Answer from the drawing. Dimensions are ordinates in mm from the lowest x, y and z of the part. Coordinates: 2 decimals unless noted, no trailing zeros. Order: outer loops, then holes, each group sorted by start corner. A loop starts at its lowest first (then second) coordinate and runs counter-clockwise, first axis right, second up. Notation, with made-up numbers: (35, -19) - (77, -19) arc R26 ccw to (77, 10) - close; hole circle Ø6 at (-33, 65). An arc over 180 degrees is marked (long way). Use a Markdown table: item, result. Add a question column.
Item 1: The part is cut by section A-A, the plane y = 63.5. Give the vertices of the cut face in (x, z), then the cut area to 3 significant figures.
Item 2: The part is cut by section B-B, the plane x = 416.5. Give the vertices of the cut face in (y, z), then the cut area to 3 significant figures.
Item 3: Find the intervals of material crossed by line 1 along Y through (x, z) = (1130, 64.5); line 2 along Z through (x, y) = (1079, 68.5); line 3 along Z through (x, y) = (1245.5, 66), in increasing order.
Item 4: Flat-ended cylindrical pins translate along their axes: P1, Ø4, axis at x = 621.5, z = 29.5, coming from the -Y side; P2, Ø5, axis at x = 978.5, y = 98.5, coming from the -Z side; P3, Ø10, axis at x = 702.5, y = 55.5, coming from the +Z side. Find the tip coordinate at first contact, or state that the pin passes through.
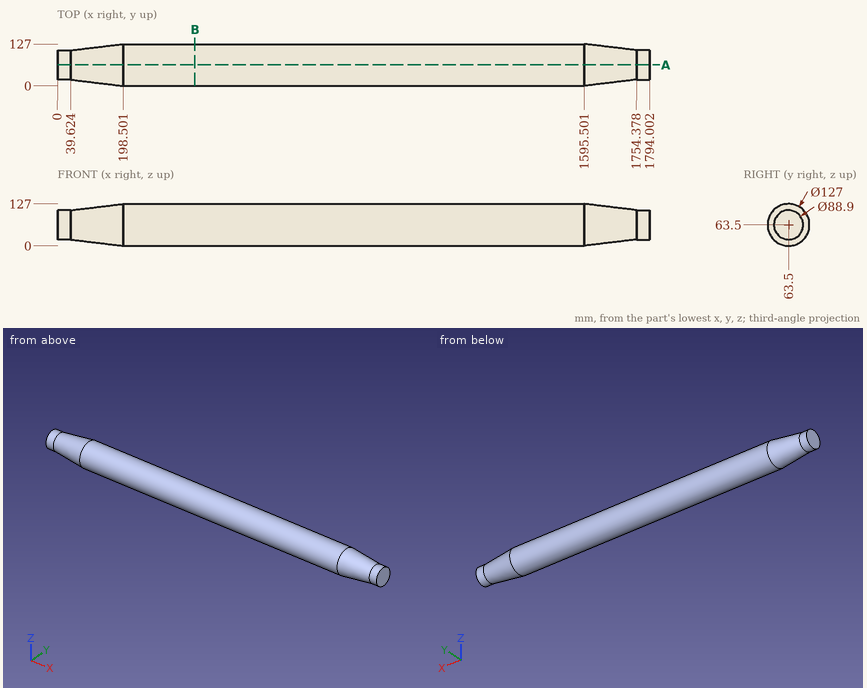
Solution:
| question | item | result |
|---|---|---|
| 1 | outline | (0, 19.05) - (39.62, 19.05) - (198.5, 0) - (1595.5, 0) - (1754.38, 19.05) - (1794, 19.05) - (1794, 107.95) - (1754.38, 107.95) - (1595.5, 127) - (198.5, 127) - (39.62, 107.95) - (0, 107.95) - close |
| 1 | area | 219,000 mm2 |
| 2 | outline | circle Ø127 at (63.5, 63.5) |
| 2 | area | 12,700 mm2 |
| 3 | line 1 | y = 0.01 to 126.99 |
| 3 | line 2 | z = 0.2 to 126.8 |
| 3 | line 3 | z = 0.05 to 126.95 |
| 4 | P1 | stops at y = 8.65 |
| 4 | P2 | stops at z = 8.95 |
| 4 | P3 | stops at z = 126.93 |
